Can you work these out from the model? Positions are in its coordinate system, mm. Coordinates: 2 decimals unless noted, no trailing zeros. Order: outer loops, then holes, each group sorted by start corner. A loop starts at its lowest first (then second) coordinate and runs counter-clockwise, first axis right, second up. Notation, with made-up numbers: (-7.75, -6) -> (42.25, -6) arc R12 cw to (42.25, 0) -> close; hole circle Ø9 at (-38.5, 78.5). An arc over 180 degrees is marked (long way). Answer as CSV lines item,"result".
from build123d import *

# Parameters (mm, degrees)
SKETCH1_R                 = 8.75
SKETCH1_R_2               = 1.5
BOSS_EXTRUDE1_DEPTH       = 5
F_2_56_TAPPED_HOLE1_D     = 1.778
F_4_40_TAPPED_HOLE1_D     = 2.2606
F_4_40_TAPPED_HOLE1_DEPTH = 7.62
F_4_40_TAPPED_HOLE1_TIP   = 0.679152758


with BuildPart() as part:
    # Sketch1 → Boss-Extrude1 (new body)
    with BuildSketch(Plane.XY):
        Circle(SKETCH1_R)
        Circle(SKETCH1_R_2, mode=Mode.SUBTRACT)
    extrude(amount=BOSS_EXTRUDE1_DEPTH)

    # #2-56 Tapped Hole1 (through all)
    with Locations(Plane.XY.offset(5)):
        with Locations((-6.35, 0), (0, 6.35), (6.35, 0), (0, -6.35)):
            Hole(F_2_56_TAPPED_HOLE1_D / 2)

    # #4-40 Tapped Hole1
    with Locations(Plane(origin=(-6.759669176, 5.556021295, 2.40860038), x_dir=(-0.634973862285, -0.772533620119, 0), z_dir=(-0.772533620119, 0.634973862285, 0))):
        with Locations((0, 0)):
            Hole(F_4_40_TAPPED_HOLE1_D / 2, depth=F_4_40_TAPPED_HOLE1_DEPTH)
            with Locations((0, 0, -(F_4_40_TAPPED_HOLE1_DEPTH + F_4_40_TAPPED_HOLE1_TIP / 2))):  # 118° drill point
                Cone(0, F_4_40_TAPPED_HOLE1_D / 2, F_4_40_TAPPED_HOLE1_TIP, mode=Mode.SUBTRACT)


solid = part.part
Q1. We'd pull the mould along X, two halves only. Please class faces 1 (the flat face through (0, -2, 0)), 2 (the cylindrical face through (4.04, -7.76, 2.46)), 3 (the cylindrical face through (7.24, 0.04, 2.46)): pulls with the +X half, pulls with the -X half, needs draft (parallel to the pull), parting line crosses it, or undercut.
Solution:
face 1,"needs draft"
face 2,"parting line crosses it"
face 3,"undercut"
Q2. Imagine slicing it at D-D (x = 2.5). List the corners of the cut face in (y, z) for me.
Solution:
outline,"(-8.39, 0) -> (8.39, 0) -> (8.39, 5) -> (-8.39, 5) -> close"
Q3. If I drill on line 1 (Y direction, x = 0, z = 3.5); line 2 (Y direction, x = -2.75, z = 2.55); line 3 (Z direction, x = -5.5, y = 5.25), over which ranges is the centre line in solid material (lowest first)?
Solution:
line 1,"-8.75 to -7.24, -5.46 to -1.5, 1.5 to 5.46, 7.24 to 8.75"
line 2,"-8.31 to 0.81, 3.71 to 8.31"
line 3,"0 to 1.43, 3.39 to 5"
Q4. Imagine slicing it at A-A (x = 6.35). List the corners of the cut face in (y, z) for me, and give its area (3 significant figures).
Solution:
outline,"(-6.02, 0) -> (-0.89, 0) -> (-0.89, 5) -> (-6.02, 5) -> close; (0.89, 0) -> (6.02, 0) -> (6.02, 5) -> (0.89, 5) -> close"
area,"51.3 mm2"
Q5. Imagine slicing it at C-C (z = 0.55). List the corners of the cut face in (x, y) for me, and give its area (3 significant figures).
Solution:
outline,"circle Ø17.5 at (0, 0); hole circle Ø1.78 at (-6.35, 0); hole circle Ø3 at (0, 0); hole circle Ø1.78 at (0, -6.35); hole circle Ø1.78 at (0, 6.35); hole circle Ø1.78 at (6.35, 0)"
area,"224 mm2"
Q6. For P1, Ø1.6, axis at x = 0, y = -6.35, coming from the -Z side; P2, Ø4, axis at x = 0, y = 0, coming from the -Z side; P3, Ø3, axis at x = 6, z = 4, coming from the +Y side, each with a flat end and sliding along its axis, tell me the tip position at first contact or that it passes through.
Solution:
P1,"through"
P2,"z = 0"
P3,"y = 7.5"
